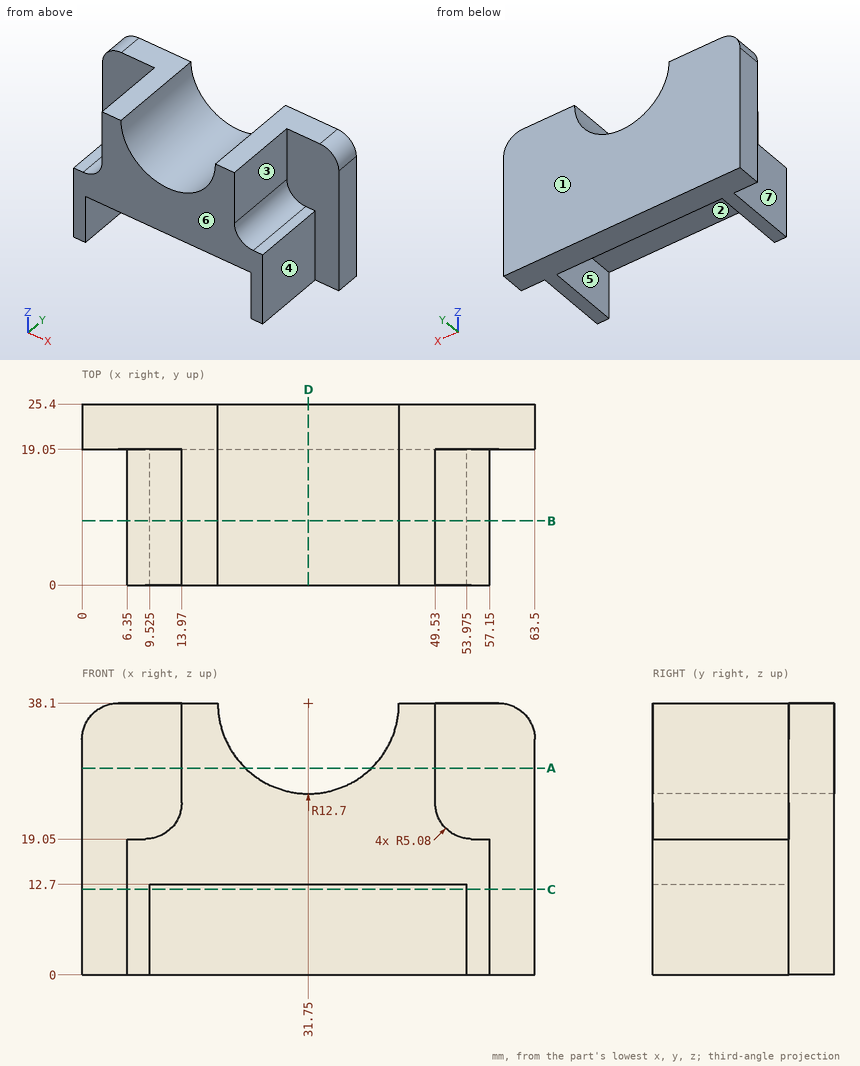
Job drawing, mm, ordinate dimensions from the low corner. One solid piece. A direction names the side the tool comes from. Give positions to 0.01 mm unless a question says otherwise; leave off trailing zeros. Loops run counter-clockwise (first coordinate to the right, second up) from the corner with the lowest first, then second, coordinate; pieces in that order, holes last. Notation, with made-up numbers: (49.25, 5) -> (107.25, 5) arc R28 ccw to (107.25, 39) -> close; hole circle Ø3 at (-9, 74.25). An arc over 180 degrees is marked (long way). Use a Markdown table: item, result. Add a question column.
(1) Slice it at C-C on z = 12. List the corners of the cut face in (x, y) (3 decimals), and give its area (3 significant figures).
(2) Slice it at B-B on y = 9. List the corners of the cut face in (x, z) (3 decimals).
(3) Slice it at A-A on z = 29. List the corners of the cut face in (x, y).
(4) Tool access for the marked faces 1, 2 and 3: list every direction of +Z, -Z, +X, -X, +Y, -Y with a clear straight run to the whole face (end or side of a thin tool).
(5) Drop flat-ended pins along their axis: pin 1 Ø4 at (y, z) = (8.5, 5) entering from -X; pin 2 Ø4 at (x, z) = (9, 11.5) entering from -Y; pin 3 Ø11 at (y, z) = (11, 33) entering from +X; pin 4 Ø4 at (y, z) = (7.5, 26.5) entering from -X. Give the stop position or say it passes through.
(6) Wall check: line 1 along X through (y, z) = (15.25, 12) (3 decimals); line 2 along Z through (x, y) = (7, 8.75); line 3 along Y through (x, z) = (61, 12.5). Give the ranges that are in metal, low to high.
(7) Slice it at D-D on x = 31.75. List the corners of the cut face in (y, z), and give its area (3 significant figures).
(8) Mould opens along X. For the marked faces 4, 5, 6 and 7 say: +X half, -X half, draft (parallel to the pull), parting line (faces both ways), or undercut.
Filled sheet:
| question | item | result |
|---|---|---|
| 1 | outline | (0, 19.05) -> (6.35, 19.05) -> (6.35, 0) -> (9.525, 0) -> (9.525, 19.05) -> (53.975, 19.05) -> (53.975, 0) -> (57.15, 0) -> (57.15, 19.05) -> (63.5, 19.05) -> (63.5, 25.4) -> (0, 25.4) -> close |
| 1 | area | 524 mm2 |
| 2 | outline | (6.35, 0) -> (9.525, 0) -> (9.525, 12.7) -> (53.975, 12.7) -> (53.975, 0) -> (57.15, 0) -> (57.15, 19.05) -> (54.61, 19.05) arc R5.08 cw to (49.53, 24.13) -> (49.53, 38.1) -> (44.45, 38.1) arc R12.7 cw to (19.05, 38.1) -> (13.97, 38.1) -> (13.97, 24.13) arc R5.08 cw to (8.89, 19.05) -> (6.35, 19.05) -> close |
| 3 | outline | (0, 19.05) -> (13.97, 19.05) -> (13.97, 0) -> (22.89, 0) -> (22.89, 25.4) -> (0, 25.4) -> close; (40.61, 0) -> (49.53, 0) -> (49.53, 19.05) -> (63.5, 19.05) -> (63.5, 25.4) -> (40.61, 25.4) -> close |
| 4 | face 1 | +Z, -Z, +X, -X, +Y |
| 4 | face 2 | -Z, -Y |
| 4 | face 3 | +Z, +X, -Y |
| 5 | pin 1 | x = 6.35 |
| 5 | pin 2 | y = 0 |
| 5 | pin 3 | x = 49.53 |
| 5 | pin 4 | x = 13.97 |
| 6 | line 1 | 6.35 to 9.525, 53.975 to 57.15 |
| 6 | line 2 | 0 to 19.05 |
| 6 | line 3 | 19.05 to 25.4 |
| 7 | outline | (0, 12.7) -> (19.05, 12.7) -> (19.05, 0) -> (25.4, 0) -> (25.4, 25.4) -> (0, 25.4) -> close |
| 7 | area | 403 mm2 |
| 8 | face 4 | +X half |
| 8 | face 5 | undercut |
| 8 | face 6 | draft |
| 8 | face 7 | -X half |
